```python
from build123d import *

# Parameters (mm, degrees)
SKETCH1_W           = 79
SKETCH1_H           = 77
BOSS_EXTRUDE1_DEPTH = 12
CUT_EXTRUDE1_DEPTH  = 37
CUT_EXTRUDE2_DEPTH  = 37
SKETCH5_W           = 28
SKETCH5_H           = 5
CUT_EXTRUDE3_DEPTH  = 77
SKETCH7_R           = 2.85
CUT_EXTRUDE5_DEPTH  = 77
SKETCH8_R           = 1.35
CUT_EXTRUDE6_DEPTH  = 4


with BuildPart() as part:
    # Sketch1 → Boss-Extrude1 (new body)
    with BuildSketch(Plane.XY):
        with Locations((39.5, 38.5)):
            Rectangle(SKETCH1_W, SKETCH1_H)
        with BuildLine():
            Line((22.86419524, 67), (56.13580476, 67))
            ThreePointArc((56.13580476, 67), (72.5, 38.5), (56.13580476, 10))
            Line((56.13580476, 10), (22.86419524, 10))
            ThreePointArc((22.86419524, 10), (6.5, 38.5), (22.86419524, 67))
        make_face(mode=Mode.SUBTRACT)
    extrude(amount=BOSS_EXTRUDE1_DEPTH)

    # Sketch3 → Cut-Extrude1 (cut)
    with BuildSketch(Plane.XZ):
        Polygon((0, 0), (1.5, 0), (1.5, 5.5), (3, 5.5), (3, 8), (0, 8), align=None)
        Polygon((79, 0), (77.5, 0), (77.5, 5.5), (76, 5.5), (76, 8), (79, 8), align=None)
    extrude(amount=-CUT_EXTRUDE1_DEPTH, mode=Mode.SUBTRACT)

    # Sketch4 → Cut-Extrude2 (cut)
    with BuildSketch(Plane(origin=(0, 77, 0), x_dir=(1, 0, 0), z_dir=(0, 1, 0))):
        Polygon((76, -8), (79, -8), (79, 0), (77.5, 0), (77.5, -5.5), (76, -5.5), align=None)
        Polygon((0, -8), (3, -8), (3, -5.5), (1.5, -5.5), (1.5, 0), (0, 0), align=None)
    extrude(amount=-CUT_EXTRUDE2_DEPTH, mode=Mode.SUBTRACT)

    # Sketch5 → Cut-Extrude3 (cut)
    with BuildSketch(Plane(origin=(0, 77, 0), x_dir=(1, 0, 0), z_dir=(0, 1, 0))):
        with Locations((58.5, -2.5)):
            Rectangle(SKETCH5_W, SKETCH5_H)
        with Locations((20.5, -2.5)):
            Rectangle(SKETCH5_W, SKETCH5_H)
    extrude(amount=-CUT_EXTRUDE3_DEPTH, mode=Mode.SUBTRACT)

    # Sketch7 → Cut-Extrude5 (cut)
    with BuildSketch(Plane.XZ):
        with Locations((39.5, 5)):
            Circle(SKETCH7_R)
    extrude(amount=-CUT_EXTRUDE5_DEPTH, mode=Mode.SUBTRACT)

    # Sketch8 → Cut-Extrude6 (cut)
    with BuildSketch(Plane.XY.offset(12)):
        with Locations((75.5, 2.5)):
            Circle(SKETCH8_R)
        with Locations((75.5, 74.5)):
            Circle(SKETCH8_R)
        with Locations((3.5, 74.5)):
            Circle(SKETCH8_R)
        with Locations((3.5, 2.5)):
            Circle(SKETCH8_R)
    extrude(amount=-CUT_EXTRUDE6_DEPTH, mode=Mode.SUBTRACT)


solid = part.part
```
The listing builds one solid part. Answer for the finished solid, in the listing's coordinates (mm). A direction names the side the tool comes from. Give positions to 0.01 mm unless a question says otherwise; leave off trailing zeros. Order: outer loops, then holes, each group sorted by start corner. A loop starts at its lowest first (then second) coordinate and runs counter-clockwise, first axis right, second up. Notation, with made-up numbers: (8, 57) - (67, 57) arc R25 ccw to (67, 84) - close; hole circle Ø9 at (-40, 32.25). An arc over 180 degrees is marked (long way). Answer in a Markdown table with one row per item. Add a question column.
Q1. The part is cut by section D-D (z = 6.5). Determine the outline of the cut face in (x, y), then the cut area to 3 significant figures.
Q2. For a pull along X with two mould halves and no side action, classify faces 1 (the cylindrical face through (42.218, 71.93, 5.856)), 2 (the flat face through (3, 59, 7)), 3 (the flat face through (79, 38, 9)), 4 (the flat face through (77, 59, 8)) as released by +X, released by -X, zero draft, split by the parting line, or undercut.
Q3. The part is cut by section A-A (x = 50). Determine the outline of the cut face in (y, z).
Q4. Which of the six approach directions +Z, -Z, +X, -X, +Y, -Y give full straight-line access (tool end or side, diameter ignored) to faces 5 (the flat face through (77.5, 18, 3)), 6 (the flat face through (75, 39, 0)), 7 (the flat face through (1.5, 59, 3)), 8 (the flat face through (17, 11, 5))?
Q5. Given P1, Ø0.8, axis at y = 13, z = 6.5, coming from the -X side; P2, Ø0.9, axis at x = 75, y = 74.5, coming from the +Z side; P3, Ø1.5, axis at y = 66, z = 3.5, coming from the -X side, each flat-ended and moving along its own axis, determine where each tip first touches the part or whether it passes through.
Q6. The part is cut by section B-B (y = 2.5). Give the number of separate pieces and of enclosed holes in the cut face, then the cut area to 3 significant figures.
Q7. The part is cut by section C-C (x = 39.5). Determine the outline of the cut face in (y, z), then the cut area to 3 significant figures.
Q8. Find the intervals of material crossed by line 1 along Y through (x, z) = (3.5, 9); line 2 along X through (y, z) = (74.5, 10.4); line 3 along X through (y, z) = (72.5, 0.75), in increasing order. Write a range as [from, to].
Determined:
| question | item | result |
|---|---|---|
| 1 | outline | (0, 37) - (3, 37) - (3, 0) - (37.08, 0) - (37.08, 10) - (22.86, 10) arc R33 cw to (22.86, 67) - (37.08, 67) - (37.08, 77) - (3, 77) - (3, 40) - (0, 40) - close; (41.92, 0) - (76, 0) - (76, 37) - (79, 37) - (79, 40) - (76, 40) - (76, 77) - (41.92, 77) - (41.92, 67) - (56.14, 67) arc R33 cw to (56.14, 10) - (41.92, 10) - close |
| 1 | area | 2,320 mm² |
| 2 | face 1 | undercut |
| 2 | face 2 | released by -X |
| 2 | face 3 | released by +X |
| 2 | face 4 | zero draft |
| 3 | outline | (0, 5) - (10, 5) - (10, 12) - (0, 12) - close; (67, 5) - (77, 5) - (77, 12) - (67, 12) - close |
| 4 | face 5 | -Z, +X, -Y |
| 4 | face 6 | -Z, +X, -X, +Y, -Y |
| 4 | face 7 | -Z, -X, +Y |
| 4 | face 8 | -Z, +Y, -Y |
| 5 | P1 | stops at x = 3 |
| 5 | P2 | stops at z = 8 |
| 5 | P3 | stops at x = 1.5 |
| 6 | separate pieces | 3 |
| 6 | enclosed holes | 1 |
| 6 | area | 589 mm² |
| 7 | outline | (0, 0) - (10, 0) - (10, 2.15) - (0, 2.15) - close; (0, 7.85) - (10, 7.85) - (10, 12) - (0, 12) - close; (67, 0) - (77, 0) - (77, 2.15) - (67, 2.15) - close; (67, 7.85) - (77, 7.85) - (77, 12) - (67, 12) - close |
| 7 | area | 126 mm² |
| 8 | line 1 | y = [0, 1.15], [3.85, 73.15], [75.85, 77] |
| 8 | line 2 | x = [0, 2.15], [4.85, 74.15], [76.85, 79] |
| 8 | line 3 | x = [1.5, 6.5], [34.5, 44.5], [72.5, 77.5] |
